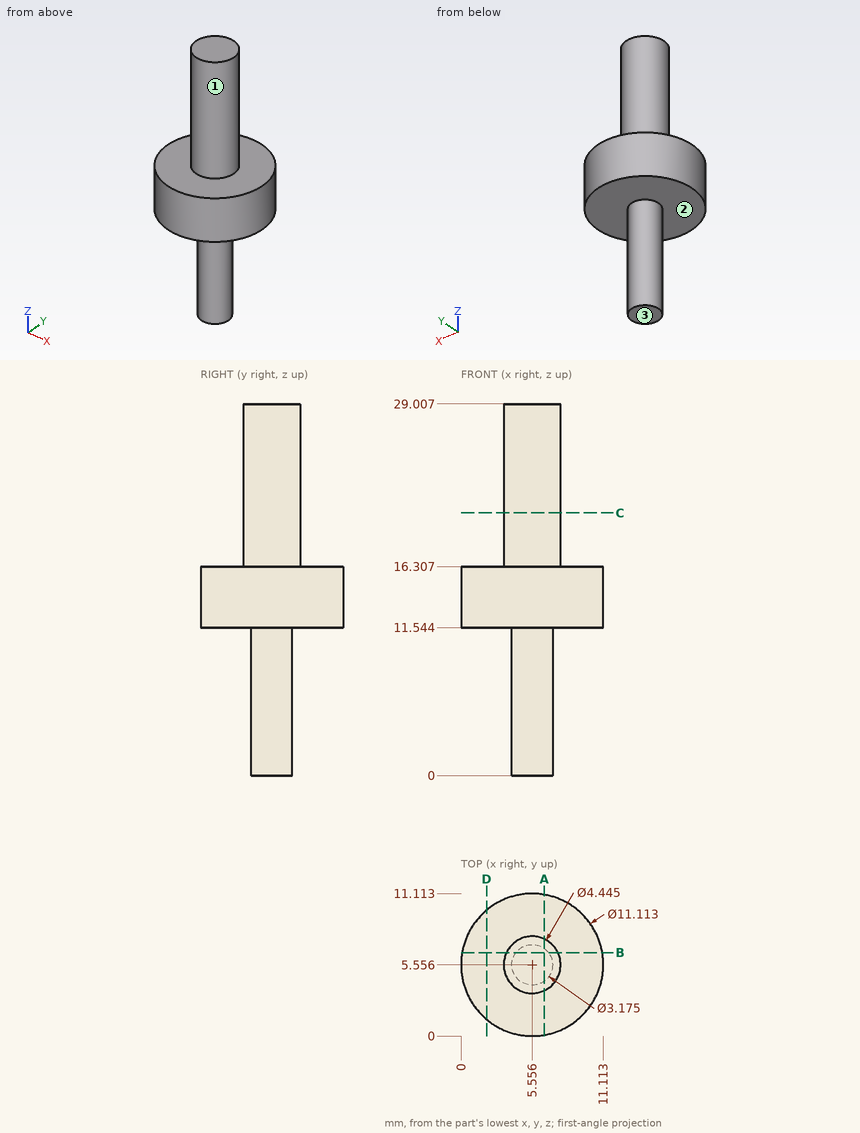
Print and shaded views of the part. All mm, measured from the part's lowest x, y and z. A direction names the side the tool comes from. Give positions to 0.01 mm unless a question says otherwise; leave off trailing zeros. Order: outer loops, then holes, each group sorted by start corner. A loop starts at its lowest first (then second) coordinate and runs counter-clockwise, first axis right, second up. Notation, with made-up numbers: (-28, 25.5) - (10, 25.5) arc R28 ccw to (10, 64.5) - close; hole circle Ø5 at (-33.5, -2.5). An arc over 180 degrees is marked (long way). Use a Markdown table: item, result.
1) 3-axis set-ups, long thin cutter, end or side, ignore diameter. For the marked faces 1, 2 and 3: which of +Z, -Z, +X, -X, +Y, -Y reach the whole face in a straight line?
Checked values:
| item | result |
|---|---|
| face 1 | +Z |
| face 2 | -Z |
| face 3 | -Z, +X, -X, +Y, -Y |
2) Probe L1, parallel to Z at x = 3.75, y = 8.25 (1 decimal); L2, parallel to Y at x = 4.5, z = 13.25; L3, parallel to Y at x = 4.25, z = 27 (1 decimal). List the from-to ranges inside material, lowest first. Write a range as from..to.
Checked values:
| item | result |
|---|---|
| L1 | 11.5..16.3 |
| L2 | 0.1..11.01 |
| L3 | 3.8..7.4 |
3) Flat gauge pins, fed straight in: P1, Ø4, axis at x = 4.5, z = 23.5, coming from the +Y side; P2, Ø1.5, axis at x = 4.5, z = 11.5, coming from the +Y side; P3, Ø4, axis at y = 6.5, z = 8.5, coming from the -X side. Where does each tip first touch, or does it go through?
Checked values:
| item | result |
|---|---|
| P1 | y = 7.78 |
| P2 | y = 11.1 |
| P3 | x = 3.97 |
4) Saw through at C-C on z = 20.5. List the corners of the cut face in (x, y) (1 decimal), plus the area to 3 significant figures.
Checked values:
| item | result |
|---|---|
| outline | circle Ø4.4 at (5.6, 5.6) |
| area | 15.5 mm² |
5) Saw through at A-A on x = 6.5. List the corners of the cut face in (y, z) (1 decimal).
Checked values:
| item | result |
|---|---|
| outline | (0.1, 11.5) - (4.3, 11.5) - (4.3, 0) - (6.8, 0) - (6.8, 11.5) - (11, 11.5) - (11, 16.3) - (7.6, 16.3) - (7.6, 29) - (3.5, 29) - (3.5, 16.3) - (0.1, 16.3) - close |
6) Saw through at D-D on x = 2. List the corners of the cut face in (y, z) (1 decimal).
Checked values:
| item | result |
|---|---|
| outline | (1.3, 11.5) - (9.8, 11.5) - (9.8, 16.3) - (1.3, 16.3) - close |
